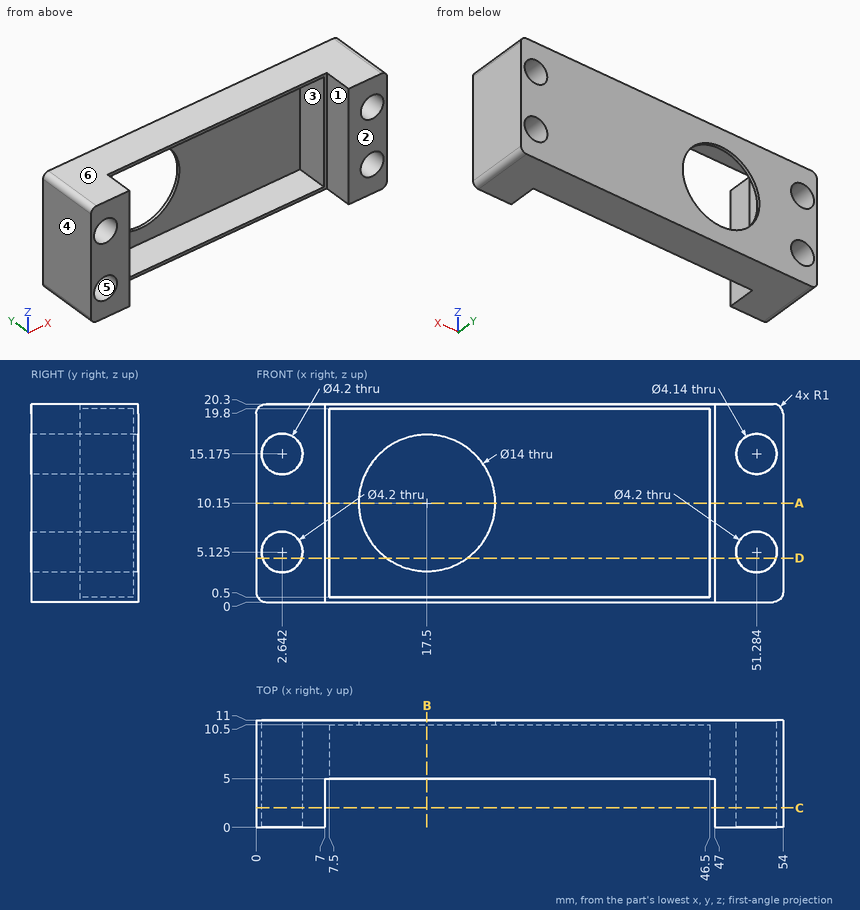
Input: dimensioned drawing with shaded views. Units: mm. Origin: part minimum x, y, z. A direction names the side the tool comes from. Give positions to 0.01 mm unless a question says otherwise; leave off trailing zeros. Write each loop counter-clockwise with the first axis right and the second up, starting at its lowest first coordinate (ties: lowest second). Pieces come first, ordered by that corner, then holes. Notation, with made-up numbers: M 24.5,-39.5 L 72.5,-39.5 A30 ccw 72.5,-11.5 Z; hole C -21,38.5 d2. An arc over 180 degrees is marked long. Return JSON: item names as keys, results as strings. Group by question number.
1) Cut plane B-B, the plane x = 17.5. Output: boundary loops of the cut face in (y, z).
2) Pin query (flat end, axial travel): P1, Ø8.5, axis at x = 17.5, z = 10.15, coming from the -Y side; P2, Ø6, axis at x = 32, z = 11, coming from the -Y side. Return the tip coordinate at first contact, or that it passes through.
3) Material intervals for line 1 along X through (y, z) = (1.75, 1.75); line 2 along X through (y, z) = (5.75, 10.25); line 3 along Z through (x, y) = (33, 9), sorted ascending. Write a range as [from, to].
4) Cut plane C-C, the plane y = 2. Output: boundary loops of the cut face in (x, z) (1 decimal).
5) Cut plane A-A, the plane z = 10.15. Output: boundary loops of the cut face in (x, y).
6) Pull-direction query (X, two-part tool) for the marked faces 4, 5 and 6; classes: pulls with the +X half, pulls with the -X half, needs draft (parallel to the pull), parting line crosses it, or undercut.
7) Set-up query: the marked faces 1, 2 and 3. Return all of +Z, -Z, +X, -X, +Y, -Y with unobstructed straight access to the full face (end or side cutting, diameter ignored); none if empty.
8) Cut plane D-D, the plane z = 4.5. Output: boundary loops of the cut face in (x, y).
Recorded:
{
 "1": {"outline": "M 5,0 L 11,0 L 11,3.15 L 10.5,3.15 L 10.5,0.5 L 5,0.5 Z; M 5,19.8 L 10.5,19.8 L 10.5,17.15 L 11,17.15 L 11,20.3 L 5,20.3 Z"},
 "2": {"P1": "passes through", "P2": "stops at y = 10.5"},
 "3": {"line 1": "x = [0, 7], [47, 54]", "line 2": "x = [0, 7.5], [46.5, 54]", "line 3": "z = [0, 0.5], [19.8, 20.3]"},
 "4": {"outline": "M 0,1 A1 ccw 1,0 L 7,0 L 7,20.3 L 1,20.3 A1 ccw 0,19.3 Z; M 47,0 L 53,0 A1 ccw 54,1 L 54,19.3 A1 ccw 53,20.3 L 47,20.3 Z; hole C 2.6,5.1 d4.2; hole C 2.6,15.2 d4.2; hole C 51.3,5.1 d4.2; hole C 51.3,15.2 d4.1"},
 "5": {"outline": "M 0,0 L 7,0 L 7,5 L 7.5,5 L 7.5,10.5 L 10.5,10.5 L 10.5,11 L 0,11 Z; M 24.5,10.5 L 46.5,10.5 L 46.5,5 L 47,5 L 47,0 L 54,0 L 54,11 L 24.5,11 Z"},
 "6": {"face 4": "pulls with the -X half", "face 5": "undercut", "face 6": "needs draft"},
 "7": {"face 1": "+Z, -Z, -Y", "face 2": "+Z, -Z, +X, -X, -Y", "face 3": "-Y"},
 "8": {"outline": "M 0,0 L 0.64,0 L 0.64,11 L 0,11 Z; M 4.65,0 L 7,0 L 7,5 L 7.5,5 L 7.5,10.5 L 13.37,10.5 L 13.37,11 L 4.65,11 Z; M 21.63,10.5 L 46.5,10.5 L 46.5,5 L 47,5 L 47,0 L 49.28,0 L 49.28,11 L 21.63,11 Z; M 53.29,0 L 54,0 L 54,11 L 53.29,11 Z"}
}
